```python
from build123d import *

# Parameters (mm, degrees)
F3_DEPTH = 22.86


with BuildPart() as f1:
    # F0 (on Top) → F1 (revolve)
    with BuildSketch(Plane.XY):
        Polygon((12.4199267048, 78.9793966675), (0, 78.9793966675), (0, -52.7196033325), (12.7, -52.7196033325), (12.7, 38.3393966675), (15.875, 41.5143966675), (15.875, 75.5243233723), align=None)
    revolve(axis=Axis((0, 13.1298966675, 0), (0, 1, 0)))

    # F2 (on Front) → F3 (join, symmetric)
    with BuildSketch(Plane.XZ):
        with BuildLine():
            Line((7.62, -11.43), (7.62, -10.16))
            ThreePointArc((7.62, -10.16), (-1.7960512242, -12.5723585695), (-10.16, -7.62))
            Line((-10.16, -7.62), (-10.16, -10.795))
            Line((-10.16, -10.795), (-20.32, -10.795))
            Line((-20.32, -10.795), (-20.32, -22.86))
            Line((-20.32, -22.86), (-8.636, -22.86))
            Line((-8.636, -22.86), (-8.636, -21.59))
            Line((-8.636, -21.59), (-10.82675, -19.39925))
            Line((-10.82675, -19.39925), (-7.9375, -16.51))
            Line((-7.9375, -16.51), (7.9375, -16.51))
            Line((7.9375, -16.51), (11.1125, -19.685))
            Line((11.1125, -19.685), (11.43, -19.685))
            Line((11.43, -19.685), (11.43, -15.24))
            Line((11.43, -15.24), (7.62, -11.43))
        make_face()
    extrude(amount=F3_DEPTH, both=True)


solid = f1.part
```
Source: CAD feature listing. Evaluate the final solid. Frame: model axes, mm. A direction names the side the tool comes from. Give positions to 0.01 mm unless a question says otherwise; leave off trailing zeros. Loops run counter-clockwise (first coordinate to the right, second up) from the corner with the lowest first, then second, coordinate; pieces in that order, holes last. Notation, with made-up numbers: (19, 22) -> (59, 22) arc R31 cw to (59, 57) -> close; hole circle Ø11 at (0, 59). An arc over 180 degrees is marked (long way). Put each result on its own line as item: value. Start each with the question number.
1) Draft query along X for faces 4 (the face through (5.86, -6.553, 11.267)), 5 (the face through (9.55, -0.32, -13.36)), 6 (the face through (0, 0, -16.51)). Return one class per face: released by +X, released by -X, zero draft, split by the parting line, or undercut.
2) Material intervals for probe 1 along Z at (x, y) = (11, 10.5); probe 2 along X at (y, z) = (57, 9.5); probe 3 along Z at (x, y) = (-18, -14) (3 decimals), sorted ascending.
3) Cut plane C-C (x = 0). Return loops of the section in (y, z) (3 decimals), then the cut area to 3 significant figures.
4) Cut plane A-A (z = 0). Return loops of the section in (x, y) (3 decimals).
5) Contact query for flat-ended pins moving along their axis: P1, Ø5, axis at x = 11.5, y = 25.5, coming from the +Z side; P2, Ø4.5, axis at x = 1, z = -16, coming from the +Y side; P3, Ø5, axis at y = -4.5, z = -17.5, coming from the +X side. Output: stop coordinate, or through.
6) Cut plane D-D (z = -18). Return loops of the section in (x, y).
7) Reachability of faces 1 (the face through (-9.4, -0.32, -17.97)), 2 (the face through (9.503, -0.32, -18.075)), 3 (the face through (-10.16, 0, -9)) from +Z, -Z, +X, -X, +Y, -Y: full face, straight path, thin tool, end or side. Return the list, or none.
Results are:
1. face 4: split by the parting line
1. face 5: released by +X
1. face 6: undercut
2. probe 1: z = -19.57 to -14.81, -6.35 to 6.35
2. probe 2: x = -12.72 to 12.72
2. probe 3: z = -22.86 to -10.795
3. outline: (-52.72, -12.7) -> (-22.86, -12.7) -> (-22.86, -16.51) -> (22.86, -16.51) -> (22.86, -12.7) -> (38.339, -12.7) -> (41.514, -15.875) -> (75.524, -15.875) -> (78.979, -12.42) -> (78.979, 12.42) -> (75.524, 15.875) -> (41.514, 15.875) -> (38.339, 12.7) -> (-52.72, 12.7) -> close
3. area: 3,760 mm2
4. outline: (-15.875, 41.514) -> (-12.7, 38.339) -> (-12.7, -52.72) -> (12.7, -52.72) -> (12.7, 38.339) -> (15.875, 41.514) -> (15.875, 75.524) -> (12.42, 78.979) -> (-12.42, 78.979) -> (-15.875, 75.524) -> close
5. P1: stops at z = 8.96
5. P2: stops at y = 77.62
5. P3: stops at x = 11.43
6. outline: (-20.32, -22.86) -> (-9.43, -22.86) -> (-9.43, 22.86) -> (-20.32, 22.86) -> close; (9.43, -22.86) -> (11.43, -22.86) -> (11.43, 22.86) -> (9.43, 22.86) -> close
7. face 1: +Y, -Y
7. face 2: -Z, +Y, -Y
7. face 3: -X, -Y
